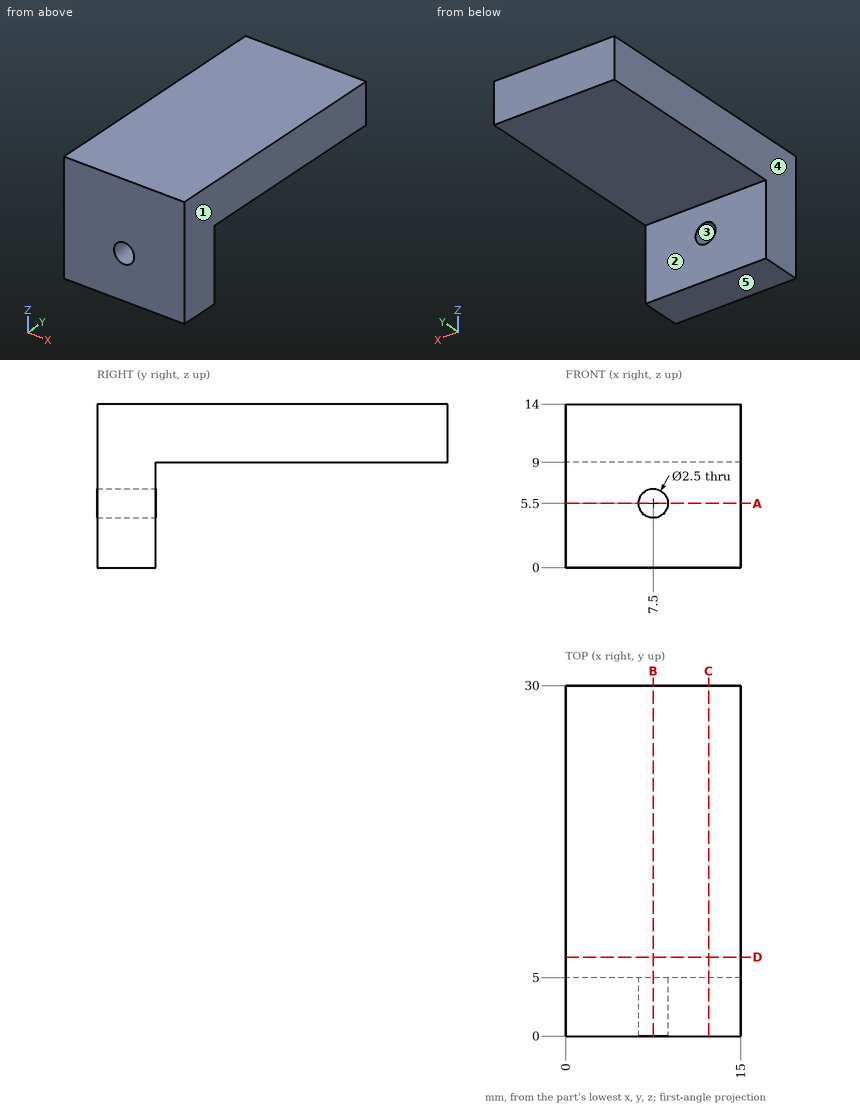
Source: three-view drawing plus pictorial views. Frame: mm from the lowest corner of the part. A direction names the side the tool comes from. Give positions to 0.01 mm unless a question says otherwise; leave off trailing zeros. Order: outer loops, then holes, each group sorted by start corner. A loop starts at its lowest first (then second) coordinate and runs counter-clockwise, first axis right, second up. Notation, with made-up numbers: M 13.5,34 L 57.5,34 A5 ccw 57.5,43 Z; hole C 56.25,45.25 d3. An arc over 180 degrees is marked long. Return JSON: item names as keys, results as strings.
Item 1: Cut plane D-D (y = 6.75). Return loops of the section in (x, z).
Solutions:
{"outline": "M 0,9 L 15,9 L 15,14 L 0,14 Z"}
Item 2: Cut plane C-C (x = 12.25). Return loops of the section in (y, z), then the cut area to 3 significant figures.
Solutions:
{"outline": "M 0,0 L 5,0 L 5,9 L 30,9 L 30,14 L 0,14 Z", "area": "195 mm^2"}
Item 3: Ray query, probe 1 along Z at (x, y) = (7.5, 2.1); probe 2 along X at (y, z) = (2.25, 5.5); probe 3 along Z at (x, y) = (6.75, 10.75). Return the intervals inside material, ascending.
Solutions:
{"probe 1": "0 to 4.25, 6.75 to 14", "probe 2": "0 to 6.25, 8.75 to 15", "probe 3": "9 to 14"}
Item 4: Access query for the marked faces 1 and 2. Directions: +Z, -Z, +X, -X, +Y, -Y. A direction counts if a zero-diameter tool reaches every point of the face in a straight line with its end or side. Return the directions, or none.
Solutions:
{"face 1": "+Z, -Z, +X, +Y, -Y", "face 2": "-Z, +X, -X, +Y"}
Item 5: Cut plane A-A (z = 5.5). Return loops of the section in (x, y), then the cut area to 3 significant figures.
Solutions:
{"outline": "M 0,0 L 6.25,0 L 6.25,5 L 0,5 Z; M 8.75,0 L 15,0 L 15,5 L 8.75,5 Z", "area": "62.5 mm^2"}
Item 6: Pull-direction query (Z, two-part tool) for the marked faces 3, 4 and 5; classes: +Z half, -Z half, draft (parallel to the pull), parting line (faces both ways), or undercut.
Solutions:
{"face 3": "undercut", "face 4": "draft", "face 5": "-Z half"}
Item 7: First-contact query: P1, Ø7, axis at x = 10.5, z = 3, coming from the +Y side; P2, Ø8, axis at x = 11, y = 14, coming from the -Z side; P3, Ø2, axis at x = 7.5, z = 5.5, coming from the -Y side. Flat tips, straight axial feed; report the tip coordinate or a pass-through.
Solutions:
{"P1": "y = 5", "P2": "z = 9", "P3": "through"}
Item 8: Cut plane B-B (x = 7.5). Return loops of the section in (y, z), then the cut area to 4 significant figures.
Solutions:
{"outline": "M 0,0 L 5,0 L 5,4.25 L 0,4.25 Z; M 0,6.75 L 5,6.75 L 5,9 L 30,9 L 30,14 L 0,14 Z", "area": "182.5 mm^2"}
